Source: CAD feature listing. Evaluate the final solid. Frame: model axes, mm. Coordinates: 2 decimals unless noted, no trailing zeros. Loops run counter-clockwise (first coordinate to the right, second up) from the corner with the lowest first, then second, coordinate; pieces in that order, holes last. Notation, with made-up numbers: M -3,64 L 55,64 A8 cw 55,72 Z; hole C 72.25,72.25 d5. An arc over 180 degrees is marked long. One line per question, with ' | ' between items. Start each with the question number.
1. Pin query (flat end, axial travel): P1, Ø1.9, axis at y = 5, z = -15.5, coming from the +X side; P2, Ø6.5, axis at x = 8, y = 50.5, coming from the +Z side; P3, Ø2, axis at y = 12, z = 9, coming from the -X side; P4, Ø3, axis at y = 3.5, z = 14.5, coming from the -X side. Return the tip coordinate at first contact, or that it passes through.
2. Section query A-A, the plane z = -1.5. Output: boundary loops of the cut face in (x, y).
3. Section query C-C, the plane z = -8. Output: boundary loops of the cut face in (x, y).
4. Section query B-B, the plane y = 13. Output: boundary loops of the cut face in (x, z).
5. Ray query, probe 1 along Y at (x, z) = (9, -16); probe 2 along Z at (x, y) = (10.5, 108); probe 3 along X at (y, z) = (45.5, -5.5). Return the intervals inside material, ascending.
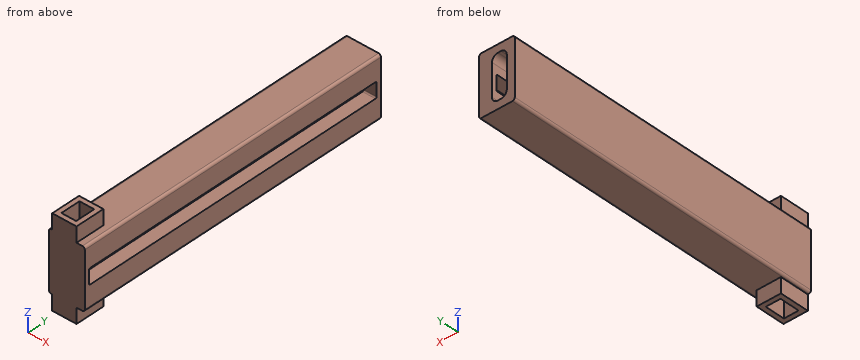
```python
from build123d import *

# Parameters (mm, degrees)
BOSS_EXTRUDE2_DEPTH  = 134
BOSS_EXTRUDE3_DEPTH  = 2
SKETCH18_W           = 5.45
SKETCH18_H           = 6.4
BOSS_EXTRUDE10_DEPTH = 2
FILLET1_R            = 0.5
FILLET2_R            = 0.5
SKETCH45_W           = 6.2
SKETCH45_H           = 8.3
CUT_EXTRUDE6_DEPTH   = 32.3
BOSS_EXTRUDE11_DEPTH = 6.3


with BuildPart() as part:
    # Sketch3 → Boss-Extrude2 (new body)
    with BuildSketch(Plane(origin=(0, 0, 0), x_dir=(1, 0, 0), z_dir=(0, 1, 0))):
        with BuildLine():
            Line((0, -11.5), (0, 11.5))
            ThreePointArc((0, 11.5), (0.292893219, 12.207106781), (1, 12.5))
            Line((1, 12.5), (14, 12.5))
            ThreePointArc((14, 12.5), (14.707106781, 12.207106781), (15, 11.5))
            Line((15, 11.5), (15, 3.2))
            Line((15, 3.2), (9.55, 3.2))
            Line((9.55, 3.2), (9.55, 6.7))
            ThreePointArc((9.55, 6.7), (8.817766953, 8.467766953), (7.05, 9.2))
            Line((7.05, 9.2), (5.85, 9.2))
            ThreePointArc((5.85, 9.2), (4.082233047, 8.467766953), (3.35, 6.7))
            Line((3.35, 6.7), (3.35, -6.7))
            ThreePointArc((3.35, -6.7), (4.082233047, -8.467766953), (5.85, -9.2))
            Line((5.85, -9.2), (7.05, -9.2))
            ThreePointArc((7.05, -9.2), (8.817766953, -8.467766953), (9.55, -6.7))
            Line((9.55, -6.7), (9.55, -3.2))
            Line((9.55, -3.2), (15, -3.2))
            Line((15, -3.2), (15, -11.5))
            ThreePointArc((15, -11.5), (14.707106781, -12.207106781), (14, -12.5))
            Line((14, -12.5), (1, -12.5))
            ThreePointArc((1, -12.5), (0.292893219, -12.207106781), (0, -11.5))
        make_face()
    extrude(amount=BOSS_EXTRUDE2_DEPTH)

    # Sketch6 → Boss-Extrude3 (add)
    with BuildSketch(Plane.XZ):
        with BuildLine():
            Line((1, 12.5), (3.35, 12.5))
            Line((3.35, 12.5), (3.35, 18.8))
            Line((3.35, 18.8), (9.55, 18.8))
            Line((9.55, 18.8), (9.55, 12.5))
            Line((9.55, 12.5), (14, 12.5))
            ThreePointArc((14, 12.5), (14.707106781, 12.207106781), (15, 11.5))
            Line((15, 11.5), (15, -11.5))
            ThreePointArc((15, -11.5), (14.707106781, -12.207106781), (14, -12.5))
            Line((14, -12.5), (9.55, -12.5))
            Line((9.55, -12.5), (9.55, -18.8))
            Line((9.55, -18.8), (3.35, -18.8))
            Line((3.35, -18.8), (3.35, -12.5))
            Line((3.35, -12.5), (1, -12.5))
            ThreePointArc((1, -12.5), (0.292893219, -12.207106781), (0, -11.5))
            Line((0, -11.5), (0, 11.5))
            ThreePointArc((0, 11.5), (0.292893219, 12.207106781), (1, 12.5))
        make_face()
    extrude(amount=BOSS_EXTRUDE3_DEPTH)

    # Sketch18 → Boss-Extrude10 (add)
    with BuildSketch(Plane(origin=(0, 134, 0), x_dir=(1, 0, 0), z_dir=(0, 1, 0))):
        with Locations((12.275, 0)):
            Rectangle(SKETCH18_W, SKETCH18_H)
    extrude(amount=-BOSS_EXTRUDE10_DEPTH)

    # Fillet1
    fillet1_edges = [part.edges().sort_by_distance(p)[0] for p in [
        (12.275, 132, 3.2),
    ]]
    fillet(fillet1_edges, radius=FILLET1_R)

    # Fillet2
    fillet2_edges = [part.edges().sort_by_distance(p)[0] for p in [
        (12.275, 132, -3.2),
        (12.275, 0, -3.2),
        (12.275, 0, 3.2),
    ]]
    fillet(fillet2_edges, radius=FILLET2_R)

    # Sketch45 → Cut-Extrude6 (cut, through all)
    with BuildSketch(Plane(origin=(0, 0, -12.5), x_dir=(-1, 0, 0), z_dir=(0, 0, -1))):
        with Locations((-6.45, 4.15)):
            Rectangle(SKETCH45_W, SKETCH45_H)
    extrude(amount=-CUT_EXTRUDE6_DEPTH, mode=Mode.SUBTRACT)

    # Sketch46 → Boss-Extrude11 (add)
    with BuildSketch(Plane(origin=(0, 0, -12.5), x_dir=(-1, 0, 0), z_dir=(0, 0, -1))):
        Polygon((-9.55, -2), (-9.55, 8.3), (-3.35, 8.3), (-3.35, -2), (-1.35, -2), (-1.35, 10.3), (-11.55, 10.3), (-11.55, -2), align=None)
    boss_extrude11 = extrude(amount=BOSS_EXTRUDE11_DEPTH)

    # Mirror1: Boss-Extrude11 across plane
    add(boss_extrude11.mirror(Plane(origin=(0, 0, 0), x_dir=(1, 0, 0), z_dir=(0, 0, -1))))


solid = part.part
```
Taken from the geometry:
1) P1: x = 11.55 | P2: z = 12.5 | P3: x = 0 | P4: x = 1.35
2) outline: M 0,-2 L 15,-2 L 15,0 L 3.35,0 L 3.35,134 L 0,134 Z; M 9.55,132 L 15,132 L 15,134 L 9.55,134 Z
3) outline: M 0,-2 L 15,-2 L 15,134 L 9.19,134 L 9.19,8.3 L 9.55,8.3 L 9.55,0 L 3.35,0 L 3.35,8.3 L 3.71,8.3 L 3.71,134 L 0,134 Z
4) outline: M 0,-11.5 A1 ccw 1,-12.5 L 14,-12.5 A1 ccw 15,-11.5 L 15,-3.2 L 9.55,-3.2 L 9.55,-6.7 A2.5 cw 7.05,-9.2 L 5.85,-9.2 A2.5 cw 3.35,-6.7 L 3.35,6.7 A2.5 cw 5.85,9.2 L 7.05,9.2 A2.5 cw 9.55,6.7 L 9.55,3.2 L 15,3.2 L 15,11.5 A1 ccw 14,12.5 L 1,12.5 A1 ccw 0,11.5 Z
5) probe 1: -2 to 0, 8.3 to 10.3 | probe 2: -12.5 to -3.2, 3.2 to 12.5 | probe 3: 0 to 3.35, 9.55 to 15
